Source: CAD feature listing. Evaluate the final solid. Frame: model axes, mm. Face numbers are marked on the shaded views. A direction names the side the tool comes from. Round coordinates to 2 decimals unless told otherwise and drop trailing zeros. Loops run counter-clockwise (first coordinate to the right, second up) from the corner with the lowest first, then second, coordinate; pieces in that order, holes last. Notation, with made-up numbers: (67.5, 82) - (102.5, 82) arc R14 ccw to (102.5, 90) - close; hole circle Ø6 at (25.5, -22). An arc over 180 degrees is marked (long way). One line per question, with ' | ' between items.
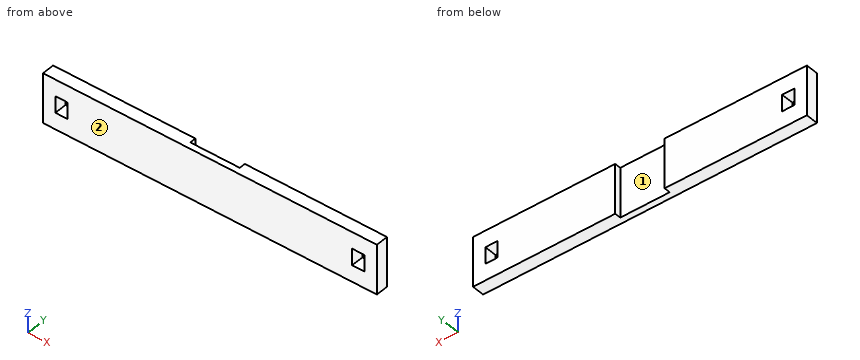
from build123d import *

# Parameters (mm, degrees)
SKETCH2_W           = 171.45
SKETCH2_H           = 25.4
BOSS_EXTRUDE1_DEPTH = 6.35
SKETCH3_W           = 6.35
SKETCH3_H           = 8.466666666
CUT_EXTRUDE1_DEPTH  = 174.437553604
SKETCH4_W           = 25.4
SKETCH4_H           = 25.4
CUT_EXTRUDE2_DEPTH  = 3.175


with BuildPart() as part:
    # Sketch2 → Boss-Extrude1 (new body)
    with BuildSketch(Plane(origin=(0, 0, 0), x_dir=(1, 0, 0), z_dir=(0, 1, 0))):
        with Locations((85.725, -12.7)):
            Rectangle(SKETCH2_W, SKETCH2_H)
    extrude(amount=BOSS_EXTRUDE1_DEPTH)

    # Sketch3 → Cut-Extrude1 (cut, through all)
    with BuildSketch(Plane(origin=(0, 6.35, 0), x_dir=(1, 0, 0), z_dir=(0, 1, 0))):
        with Locations((161.925, -12.7)):
            Rectangle(SKETCH3_W, SKETCH3_H)
        with Locations((9.525, -12.7)):
            Rectangle(SKETCH3_W, SKETCH3_H)
    extrude(amount=-CUT_EXTRUDE1_DEPTH, mode=Mode.SUBTRACT)

    # Sketch4 → Cut-Extrude2 (cut)
    with BuildSketch(Plane(origin=(0, 6.35, 0), x_dir=(1, 0, 0), z_dir=(0, 1, 0))):
        with Locations((85.725, -12.7)):
            Rectangle(SKETCH4_W, SKETCH4_H)
    extrude(amount=-CUT_EXTRUDE2_DEPTH, mode=Mode.SUBTRACT)


solid = part.part
1. Section query C-C, the plane x = 87. Return loops of the section in (y, z) (3 decimals), plus the area to 3 significant figures.
Worked out:
outline: (0, 0) - (3.175, 0) - (3.175, 25.4) - (0, 25.4) - close | area: 80.6 mm2
2. Material intervals for probe 1 along X at (y, z) = (3.25, 9.25) (3 decimals); probe 2 along X at (y, z) = (2, 13.5); probe 3 along X at (y, z) = (5.5, 8.25) (3 decimals), sorted ascending.
Worked out:
probe 1: x = 0 to 6.35, 12.7 to 73.025, 98.425 to 158.75, 165.1 to 171.45 | probe 2: x = 0 to 6.35, 12.7 to 158.75, 165.1 to 171.45 | probe 3: x = 0 to 73.025, 98.425 to 171.45
3. Section query B-B, the plane z = 23. Return loops of the section in (x, y) (3 decimals).
Worked out:
outline: (0, 0) - (171.45, 0) - (171.45, 6.35) - (98.425, 6.35) - (98.425, 3.175) - (73.025, 3.175) - (73.025, 6.35) - (0, 6.35) - close
4. Contact query for a flat-ended pin moving along its axis: P1, Ø12.5, axis at x = 84, z = 12.5, coming from the +Y side (3 decimals). Output: stop coordinate, or through.
Worked out:
P1: stops at y = 3.175
5. Access query for the marked faces 1 and 2. Directions: +Z, -Z, +X, -X, +Y, -Y. A direction counts if a zero-diameter tool reaches every point of the face in a straight line with its end or side. Return the directions, or none.
Worked out:
face 1: +Z, -Z, +Y | face 2: +Z, -Z, +X, -X, -Y
6. Section query A-A, the plane y = 5. Return loops of the section in (x, z) (3 decimals), plus the area to 3 significant figures.
Worked out:
outline: (0, 0) - (73.025, 0) - (73.025, 25.4) - (0, 25.4) - close; (98.425, 0) - (171.45, 0) - (171.45, 25.4) - (98.425, 25.4) - close; hole (6.35, 8.467) - (12.7, 8.467) - (12.7, 16.933) - (6.35, 16.933) - close; hole (158.75, 8.467) - (165.1, 8.467) - (165.1, 16.933) - (158.75, 16.933) - close | area: 3,600 mm2
